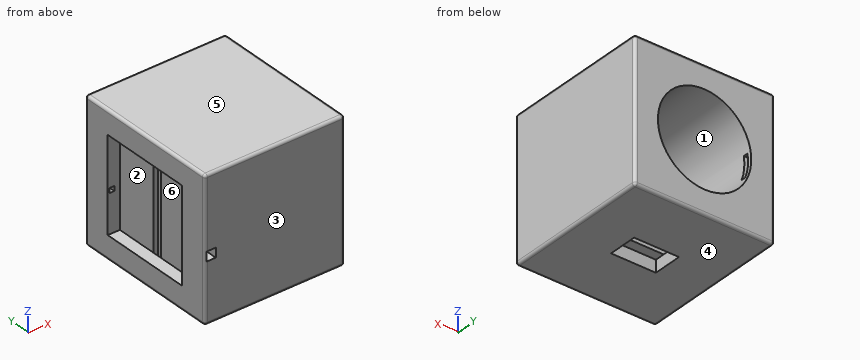
```python
from build123d import *

# Parameters (mm, degrees)
SKETCH6_W               = 150
SKETCH6_H               = 150
SKETCH6_R               = 50
BOSS_EXTRUDE4_DEPTH     = 150
SKETCH7_W               = 150
SKETCH7_H               = 150
BOSS_EXTRUDE5_DEPTH     = 10
SKETCH8_W               = 5
SKETCH8_H               = 10
CUT_EXTRUDE4_DEPTH      = 226
CUT_EXTRUDE5_DEPTH      = 226
CUT_EXTRUDE5_DEPTH_BACK = 226
SKETCH9_W               = 5
SKETCH9_H               = 10
CUT_EXTRUDE6_DEPTH      = 226
CUT_EXTRUDE6_DEPTH_BACK = 13
SKETCH10_W              = 48
SKETCH10_H              = 31
FILLET2_R               = 3
SKETCH18_W              = 100
SKETCH18_H              = 100
CUT_EXTRUDE10_DEPTH     = 13
SKETCH19_W              = 10
SKETCH19_H              = 10
CUT_EXTRUDE11_DEPTH     = 35
SKETCH21_W              = 5
SKETCH21_H              = 5
CUT_EXTRUDE12_DEPTH     = 25.72
SKETCH23_W              = 25
SKETCH23_H              = 5
CUT_EXTRUDE13_DEPTH     = 28
SKETCH24_W              = 5
SKETCH24_H              = 10
BOSS_EXTRUDE6_DEPTH     = 2
SKETCH27_W              = 5
SKETCH27_H              = 10
BOSS_EXTRUDE8_DEPTH     = 2
SKETCH31_W              = 5
SKETCH31_H              = 10
BOSS_EXTRUDE12_DEPTH    = 2
SKETCH32_W              = 5
SKETCH32_H              = 10
BOSS_EXTRUDE13_DEPTH    = 2


with BuildPart() as part:
    # Sketch6 → Boss-Extrude4 (new body)
    with BuildSketch(Plane(origin=(0, 0, 0), x_dir=(1, 0, 0), z_dir=(0, 1, 0))):
        Rectangle(SKETCH6_W, SKETCH6_H)
        with Locations(Location((0, 0, 0), (0, 0, 270))):
            Circle(SKETCH6_R, mode=Mode.SUBTRACT)
    extrude(amount=BOSS_EXTRUDE4_DEPTH)

    # Sketch7 → Boss-Extrude5 (add)
    with BuildSketch(Plane.XZ):
        Rectangle(SKETCH7_W, SKETCH7_H)
    extrude(amount=BOSS_EXTRUDE5_DEPTH)

    # Sketch8 → Cut-Extrude4 (cut, symmetric)
    with BuildSketch(Plane.XY.offset(75)):
        with Locations((59.5, 70)):
            Rectangle(SKETCH8_W, SKETCH8_H)
    cut_extrude4 = extrude(amount=CUT_EXTRUDE4_DEPTH, both=True, mode=Mode.SUBTRACT)

    # Mirror4: Cut-Extrude4 across plane
    add(cut_extrude4.mirror(Plane(origin=(0, 0, 0), x_dir=(0, 0, 1), z_dir=(1, 0, 0))), mode=Mode.SUBTRACT)

    # Sketch9 → Cut-Extrude5 (cut, two sides: drawn at the far end of the back side and taken through both)
    with BuildSketch(Plane(origin=(75, 0, 0), x_dir=(0, 0, -1), z_dir=(1, 0, 0)).offset(-CUT_EXTRUDE5_DEPTH_BACK)):
        with Locations((59.5, 70)):
            Rectangle(SKETCH9_W, SKETCH9_H)
    extrude(amount=CUT_EXTRUDE5_DEPTH + CUT_EXTRUDE5_DEPTH_BACK, mode=Mode.SUBTRACT)

    # Sketch10 → Cut-Extrude6 (cut, two sides: drawn at the far end of the back side and taken through both)
    with BuildSketch(Plane(origin=(0, 0, -75), x_dir=(-1, 0, 0), z_dir=(0, 0, -1)).offset(-CUT_EXTRUDE6_DEPTH_BACK)):
        with Locations((0, 70)):
            Rectangle(SKETCH10_W, SKETCH10_H)
    extrude(amount=CUT_EXTRUDE6_DEPTH + CUT_EXTRUDE6_DEPTH_BACK, mode=Mode.SUBTRACT)

    # Fillet2
    fillet2_edges = [part.edges().sort_by_distance(p)[0] for p in [
        (-75, 150, 0),
        (0, 150, 75),
        (0, -10, -75),
        (75, -10, 0),
        (0, -10, 75),
        (-75, -10, 0),
        (75, 150, 0),
        (75, 70, 75),
        (-75, 70, 75),
        (-75, 70, -75),
        (75, 70, -75),
        (0, 150, -75),
    ]]
    fillet(fillet2_edges, radius=FILLET2_R)

    # Sketch18 → Cut-Extrude10 (cut)
    with BuildSketch(Plane.ZY.offset(75)):
        with Locations((0, 70)):
            Rectangle(SKETCH18_W, SKETCH18_H)
    extrude(amount=-CUT_EXTRUDE10_DEPTH, mode=Mode.SUBTRACT)

    # Sketch19 → Cut-Extrude11 (cut)
    with BuildSketch(Plane(origin=(0, 20, 0), x_dir=(1, 0, 0), z_dir=(0, 1, 0))):
        with Locations((-68, 6.512866789)):
            Rectangle(SKETCH19_W, SKETCH19_H)
    extrude(amount=-CUT_EXTRUDE11_DEPTH, mode=Mode.SUBTRACT)

    # Sketch21 → Cut-Extrude12 (cut)
    with BuildSketch(Plane.XZ.offset(-120)):
        with Locations((-70.5, -6.339504826)):
            Rectangle(SKETCH21_W, SKETCH21_H)
    extrude(amount=-CUT_EXTRUDE12_DEPTH, mode=Mode.SUBTRACT)

    # Sketch23 → Cut-Extrude13 (cut)
    with BuildSketch(Plane.ZY.offset(42)):
        with Locations((-4.5, 143.222196011)):
            Rectangle(SKETCH23_W, SKETCH23_H)
    extrude(amount=CUT_EXTRUDE13_DEPTH, mode=Mode.SUBTRACT)

    # Sketch24 → Boss-Extrude6 (add)
    with BuildSketch(Plane.XY.offset(75)):
        with Locations((-59.5, 70)):
            Rectangle(SKETCH24_W, SKETCH24_H)
        with Locations((59.5, 70)):
            Rectangle(SKETCH24_W, SKETCH24_H)
    extrude(amount=-BOSS_EXTRUDE6_DEPTH)

    # Sketch27 → Boss-Extrude8 (add)
    with BuildSketch(Plane(origin=(0, 0, -75), x_dir=(-1, 0, 0), z_dir=(0, 0, -1))):
        with Locations((59.5, 70)):
            Rectangle(SKETCH27_W, SKETCH27_H)
        with Locations((-59.5, 70)):
            Rectangle(SKETCH27_W, SKETCH27_H)
    extrude(amount=-BOSS_EXTRUDE8_DEPTH)

    # Sketch31 → Boss-Extrude12 (add)
    with BuildSketch(Plane(origin=(75, 0, 0), x_dir=(0, 0, -1), z_dir=(1, 0, 0))):
        with Locations((59.5, 70)):
            Rectangle(SKETCH31_W, SKETCH31_H)
    extrude(amount=-BOSS_EXTRUDE12_DEPTH)

    # Sketch32 → Boss-Extrude13 (add)
    with BuildSketch(Plane.ZY.offset(75)):
        with Locations((-59.5, 70)):
            Rectangle(SKETCH32_W, SKETCH32_H)
    extrude(amount=-BOSS_EXTRUDE13_DEPTH)


solid = part.part
```
Input: part model. Units: mm. Frame: model coordinates. Face numbers are marked on the shaded views. A direction names the side the tool comes from. Round coordinates to 2 decimals unless told otherwise and drop trailing zeros. Order: outer loops, then holes, each group sorted by start corner. A loop starts at its lowest first (then second) coordinate and runs counter-clockwise, first axis right, second up. Notation, with made-up numbers: (-22.75, 16) - (7.25, 16) arc R18 ccw to (7.25, 39) - close; hole circle Ø9 at (70, 64.5). An arc over 180 degrees is marked (long way). One line per question, with ' | ' between items. Start each with the question number.
1) Cut plane B-B, the plane y = 29.5. Return the cut outline in (x, z), then the cut area to 3 significant figures.
2) Cut plane A-A, the plane x = -59.5. Return the cut outline in (y, z), then the cut area to 3 significant figures.
3) Ray query, probe 1 along X at (y, z) = (73, 0); probe 2 along X at (y, z) = (84, 0); probe 3 along X at (y, z) = (66, 37.5). Return the intervals inside material, ascending.
4) Cut plane C-C, the plane z = -32.5. Return the cut outline in (x, y), then the cut area to 3 significant figures.
5) Pull-direction query (Z, two-part tool) for the marked faces 4, 5 and 6; classes: +Z half, -Z half, draft (parallel to the pull), parting line (faces both ways), or undercut.
6) Set-up query: the marked faces 1, 2 and 3. Return all of +Z, -Z, +X, -X, +Y, -Y with unobstructed straight access to the full face (end or side cutting, diameter ignored); none if empty.
7) Cut plane D-D, the plane x = 0. Return the cut outline in (y, z), then the cut area to 3 significant figures.
8) Contact query for flat-ended pins moving along their axis: P1, Ø1.5, axis at y = 93, z = 16, coming from the -X side; P2, Ø5, axis at x = 0.5, y = 58, coming from the -Z side; P3, Ø12, axis at x = 2.5, z = 8.5, coming from the +Y side. Output: stop coordinate, or through.
Worked out:
1) outline: (-75, -72) arc R3 ccw to (-72, -75) - (72, -75) arc R3 ccw to (75, -72) - (75, 72) arc R3 ccw to (72, 75) - (-72, 75) arc R3 ccw to (-75, 72) - (-75, 50) - (-62, 50) - (-62, -50) - (-75, -50) - close; hole circle Ø100 at (0, 0) | area: 13,300 mm^2
2) outline: (-10, -72) arc R3 ccw to (-7, -75) - (147, -75) arc R3 ccw to (150, -72) - (150, 72) arc R3 ccw to (147, 75) - (-7, 75) arc R3 ccw to (-10, 72) - close; hole (65, -73) - (75, -73) - (75, 73) - (65, 73) - close; hole (140.72, -17) - (145.72, -17) - (145.72, 8) - (140.72, 8) - close | area: 22,400 mm^2
3) probe 1: x = -57 to -50, 50 to 57, 62 to 75 | probe 2: x = -62 to -50, 50 to 75 | probe 3: x = -57 to -33.07, 33.07 to 57, 62 to 75
4) outline: (-75, -7) arc R3 ccw to (-72, -10) - (72, -10) arc R3 ccw to (75, -7) - (75, 147) arc R3 ccw to (72, 150) - (38, 150) - (38, 0) - (-38, 0) - (-38, 150) - (-72, 150) arc R3 ccw to (-75, 147) - (-75, 120) - (-62, 120) - (-62, 75) - (-57, 75) - (-57, 65) - (-62, 65) - (-62, 20) - (-75, 20) - close; hole (57, 65) - (62, 65) - (62, 75) - (57, 75) - close | area: 11,200 mm^2
5) face 4: -Z half | face 5: +Z half | face 6: undercut
6) face 1: +Y | face 2: -X | face 3: +Z, -Z, +X, -X, -Y
7) outline: (-10, -72) arc R3 ccw to (-7, -75) - (54.5, -75) - (54.5, -62) - (65, -62) - (65, -57) - (75, -57) - (75, -62) - (85.5, -62) - (85.5, -75) - (147, -75) arc R3 ccw to (150, -72) - (150, -50) - (0, -50) - (0, 50) - (150, 50) - (150, 72) arc R3 ccw to (147, 75) - (-7, 75) arc R3 ccw to (-10, 72) - close | area: 8,540 mm^2
8) P1: stops at x = -62 | P2: stops at z = -62 | P3: stops at y = 0
